For this review, take the finished solid that the model builds, in its own axes (mm). Face numbers are marked on the shaded views. A direction names the side the tool comes from. Coordinates: 2 decimals unless noted, no trailing zeros. Loops run counter-clockwise (first coordinate to the right, second up) from the corner with the lowest first, then second, coordinate; pieces in that order, holes last. Notation, with made-up numbers: M 79.25,-9 L 126.25,-9 A15 cw 126.25,1 Z; hole C -32,0.25 d8. An arc over 180 degrees is marked long. Answer as a JSON object with one key per item and string values. Group by question number.
Item 1: Mouldability with a two-part tool opening along X and no side actions: class the marked faces 4, 5 and 6 as +X half, -X half, draft (parallel to the pull), parting line (faces both ways), or undercut.
Item 2: Add section D-D (z = 38.5). State the section outline as (x, y) points.
Item 3: Add section A-A (x = 1). State the section outline as (y, z) points.
Item 4: Tool access review of the marked faces 1, 2 and 3: name each direction out of +Z, -Z, +X, -X, +Y, -Y from which nothing blocks a thin tool from reaching the whole face with its end or side.
Item 5: Insertion check: pin 1 (1.5 mm diameter, centred on y = 5, z = 61, fed in from +X); pin 2 (3 mm diameter, centred on y = -70.5, z = 41, fed in from -X); pin 3 (3 mm diameter, centred on y = -35.5, z = 50, fed in from +X); pin 4 (20.5 mm diameter, centred on y = -17.5, z = 14, fed in from -X). Each pin has a flat end and moves straight along its axis. Give the tip position at first contact, or say it passes through.
Item 6: Wall thickness on L1, parallel to X at y = -13, z = 27; L2, parallel to Z at x = -168, y = 15; L3, parallel to Y at x = 6.5, z = 48: over which ranges is each line inside the solid? List them lowest first. Write a range as from..to.
Item 7: Add section B-B (z = -41). State the section outline as (x, y) points, then the cut area to 3 significant figures.
Item 8: Add section C-C (x = -178). State the section outline as (y, z) points.
from build123d import *

# Parameters (mm, degrees)
F1_DEPTH      = 25.4
F2_R          = 76.2
F3_DEPTH      = 76.2
F3_DEPTH_BACK = 50.8
F5_R          = 68.0716373703
F6_DEPTH      = 114.3


with BuildPart() as f1:
    # F0 (on Front) → F1 (new body)
    with BuildSketch(Plane.XZ):
        Polygon((34.8995993793, 49.2647366976), (-41.3004006207, 49.2647366976), (-41.3004006207, 23.8647366976), (9.4995993793, 23.8647366976), (9.4995993793, -1.5352633024), (-41.3004006207, -1.5352633024), (-41.3004006207, -26.9352633024), (34.8995993793, -26.9352633024), align=None)
    extrude(amount=F1_DEPTH)

    # F2 (on Top) → F3 (join, two sides)
    with BuildSketch(Plane.XY) as f3_sk:
        with Locations((-116.4346138661, -12.7)):
            Circle(F2_R)
    extrude(amount=F3_DEPTH)
    extrude(f3_sk.sketch, amount=-F3_DEPTH_BACK)

    # F5 (on face) → F6 (cut)
    with BuildSketch(Plane.XY.offset(76.2)):
        with Locations((-116.2916272879, -13.451478444)):
            Circle(F5_R)
    extrude(amount=-F6_DEPTH, mode=Mode.SUBTRACT)


solid = f1.part
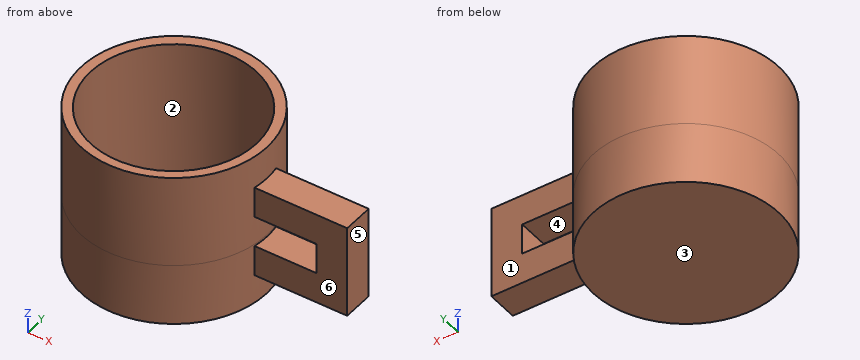
From the geometry:
{
 "1": {"face 4": "undercut", "face 5": "+X half", "face 6": "draft"},
 "2": {"outline": "M -41.3,-25.4 L 34.9,-25.4 L 34.9,0 L -41.3,0 A76.2 ccw long Z; hole C -116.29,-13.45 d136.14"},
 "3": {"outline": "M -25.4,-26.94 L 0,-26.94 L 0,-1.54 L -25.4,-1.54 Z; M -25.4,23.86 L 0,23.86 L 0,49.26 L -25.4,49.26 Z"},
 "4": {"face 1": "+Z, -Z, +X, +Y", "face 2": "+Z", "face 3": "-Z, +X, -X, +Y, -Y"},
 "5": {"pin 1": "stops at x = -42.14", "pin 2": "stops at x = -167.78", "pin 3": "stops at x = -43.27", "pin 4": "stops at x = -192.63"},
 "6": {"L1": "x = -192.63..-184.36, -48.22..34.9", "L2": "z = -50.8..-38.1", "L3": "y = -25.4..0"},
 "7": {"outline": "C -116.43,-12.7 d152.4", "area": "18,200 mm²"},
 "8": {"outline": "M -57.6,-50.8 L 32.2,-50.8 L 32.2,76.2 L 15.29,76.2 L 15.29,-38.1 L -42.19,-38.1 L -42.19,76.2 L -57.6,76.2 Z"}
}
